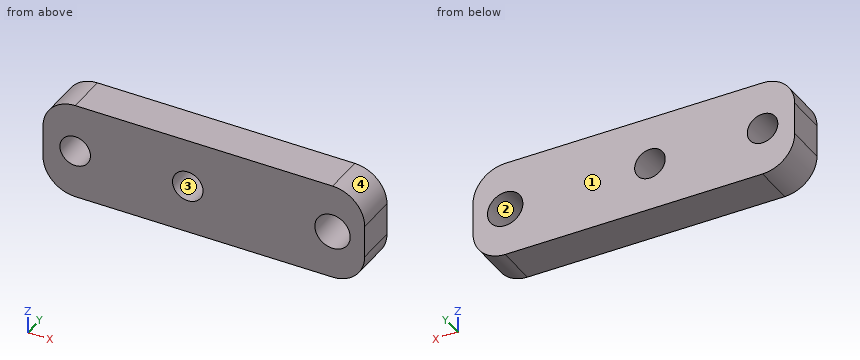
from build123d import *

# Parameters (mm, degrees)
SKETCH_1_W          = 20
SKETCH_1_H          = 6
EXTRUDE_1_DEPTH     = 2.5
SKETCH_2_R          = 1.1
SKETCH_2_R_2        = 0.95
CUT_EXTRUDE_1_DEPTH = 31.72599184
FILLET_1_R          = 2


with BuildPart() as part:
    # 草图1 → 凸台-拉伸1 (new body)
    with BuildSketch(Plane(origin=(0, 0, 0), x_dir=(1, 0, 0), z_dir=(0, 1, 0))):
        with Locations((20.030593976, 3)):
            Rectangle(SKETCH_1_W, SKETCH_1_H)
    extrude(amount=EXTRUDE_1_DEPTH)

    # 草图2 → 切除-拉伸1 (cut, through all)
    with BuildSketch(Plane(origin=(0, 2.5, 0), x_dir=(1, 0, 0), z_dir=(0, 1, 0))):
        with Locations(Location((28.030593976, 3, 0), (0, 0, 270))):
            Circle(SKETCH_2_R)
        with Locations(Location((12.030593976, 3, 0), (0, 0, 270))):
            Circle(SKETCH_2_R_2)
        with Locations(Location((19.030593976, 3, 0), (0, 0, 270))):
            Circle(SKETCH_2_R_2)
    extrude(amount=-CUT_EXTRUDE_1_DEPTH, mode=Mode.SUBTRACT)

    # 圆角1
    fillet_1_edges = [part.edges().sort_by_distance(p)[0] for p in [
        (10.030593976, 1.25, -6),
        (30.030593976, 1.25, -6),
        (30.030593976, 1.25, 0),
        (10.030593976, 1.25, 0),
    ]]
    fillet(fillet_1_edges, radius=FILLET_1_R)


solid = part.part
The model under review builds one solid part; all positions refer to its coordinate system, in mm. Face numbers are marked on the shaded views. Round coordinates to 2 decimals unless told otherwise and drop trailing zeros. Write each loop counter-clockwise with the first axis right and the second up, starting at its lowest first coordinate (ties: lowest second). Pieces come first, ordered by that corner, then holes. Notation, with made-up numbers: M 71.5,-39 L 103.5,-39 A20 ccw 103.5,-3 Z; hole C 77,13 d4. An arc over 180 degrees is marked long. Answer as CSV lines item,"result". Start each with the question number.
Q1. Consider section B-B, the plane x = 27.5. Give the boundary of the cut face in (y, z).
Q2. The part is to be moulded in two halves that separate along Z. For the marked faces 1, 2, 3 and 4, say which applies: +Z half, -Z half, draft (parallel to the pull), parting line (faces both ways), or undercut.
Q3. Consider section C-C, the plane y = 1.2. Give the boundary of the cut face in (x, z).
Q4. Clearance check with a flat-ended pin moving along its axis: P1, Ø2, axis at x = 28.03, z = -3, coming from the -Y side. State where the tip first meets the part, or that it passes through.
Q5. Consider section D-D, the plane z = -1. Give the boundary of the cut face in (x, y).
Q6. Consider section A-A, the plane z = -3. Give the boundary of the cut face in (x, y), then the cut area to 3 significant figures.
Q7. Wall thickness on line 1 along X through (y, z) = (1.05, -3); line 2 along X through (y, z) = (0.8, -3.8); line 3 along Z through (x, y) = (19.75, 0.9): over which ranges is each line inside the solid? List them lowest first.
Result set:
1,outline,"M 0,-6 L 2.5,-6 L 2.5,-3.96 L 0,-3.96 Z; M 0,-2.04 L 2.5,-2.04 L 2.5,0 L 0,0 Z"
2,face 1,"draft"
2,face 2,"undercut"
2,face 3,"undercut"
2,face 4,"+Z half"
3,outline,"M 10.03,-4 A2 ccw 12.03,-6 L 28.03,-6 A2 ccw 30.03,-4 L 30.03,-2 A2 ccw 28.03,0 L 12.03,0 A2 ccw 10.03,-2 Z; hole C 12.03,-3 d1.9; hole C 19.03,-3 d1.9; hole C 28.03,-3 d2.2"
4,P1,"passes through"
5,outline,"M 10.3,0 L 29.76,0 L 29.76,2.5 L 10.3,2.5 Z"
6,outline,"M 10.03,0 L 11.08,0 L 11.08,2.5 L 10.03,2.5 Z; M 12.98,0 L 18.08,0 L 18.08,2.5 L 12.98,2.5 Z; M 19.98,0 L 26.93,0 L 26.93,2.5 L 19.98,2.5 Z; M 29.13,0 L 30.03,0 L 30.03,2.5 L 29.13,2.5 Z"
6,area,"35.0 mm²"
7,line 1,"x = 10.03 to 11.08, 12.98 to 18.08, 19.98 to 26.93, 29.13 to 30.03"
7,line 2,"x = 10.03 to 11.52, 12.54 to 18.52, 19.54 to 27.28, 28.79 to 30.03"
7,line 3,"z = -6 to -3.62, -2.38 to 0"
